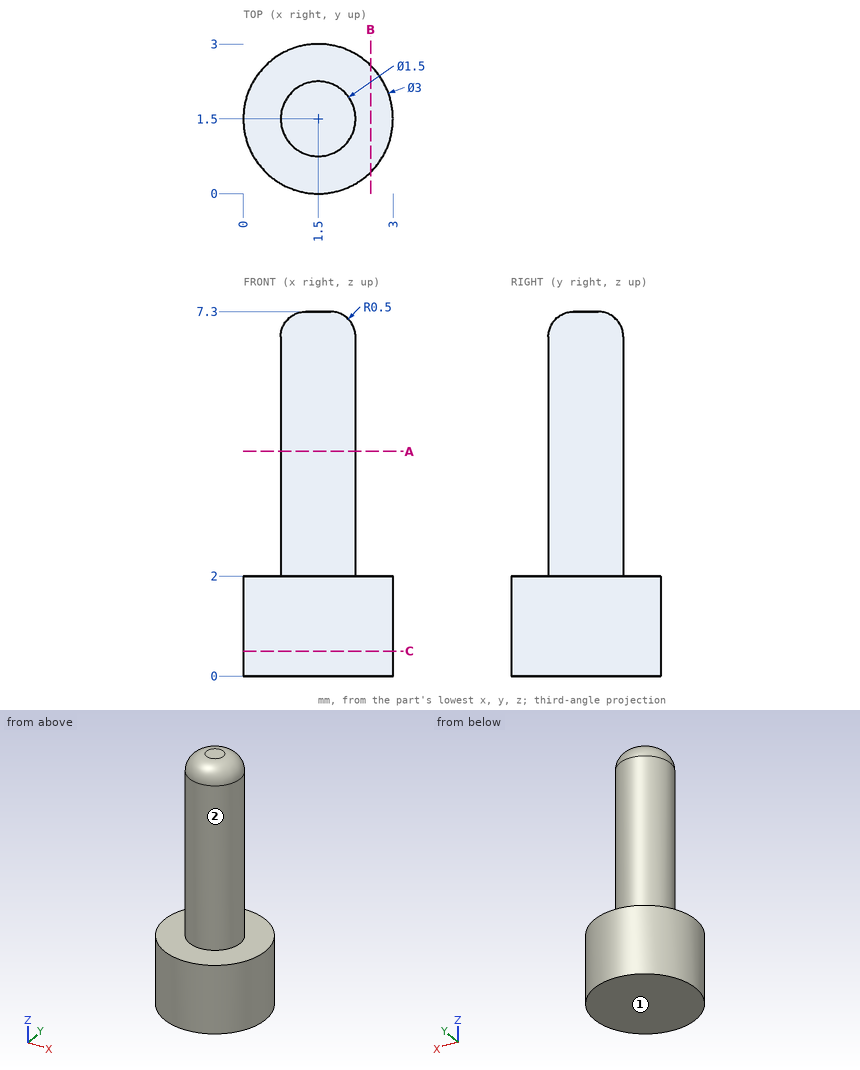
The drawing under review shows one solid part. Ordinate dimensions are in mm from its lowest x, y, z. A direction names the side the tool comes from. Give positions to 0.01 mm unless a question says otherwise; leave off trailing zeros. Write each loop counter-clockwise with the first axis right and the second up, starting at its lowest first coordinate (ties: lowest second). Pieces come first, ordered by that corner, then holes.
1. Wall thickness on L1, parallel to Z at x = 2.1, y = 0.2; L2, parallel to Y at x = 1.5, z = 3.75; L3, parallel to X at y = 2.55, z = 1.75: over which ranges is each line inside the solid? List them lowest first.
2. Add section B-B, the plane x = 2.55. Write out the cut boundary in (y, z).
3. For P1, Ø1, axis at y = 1.5, z = 6.5, coming from the -X side, flat-tipped, find the tip position at first contact; note if it passes through.
4. Add section C-C, the plane z = 0.5. Write out the cut boundary in (x, y).
5. Add section A-A, the plane z = 4.5. Write out the cut boundary in (x, y).
6. Tool access review of the marked faces 1 and 2: name each direction out of +Z, -Z, +X, -X, +Y, -Y from which nothing blocks a thin tool from reaching the whole face with its end or side.
Worked answers:
1. L1: z = 0 to 2
1. L2: y = 0.75 to 2.25
1. L3: x = 0.43 to 2.57
2. outline: (0.43, 0) - (2.57, 0) - (2.57, 2) - (0.43, 2) - close
3. P1: stops at x = 0.75
4. outline: circle Ø3 at (1.5, 1.5)
5. outline: circle Ø1.5 at (1.5, 1.5)
6. face 1: -Z, +X, -X, +Y, -Y
6. face 2: +Z
